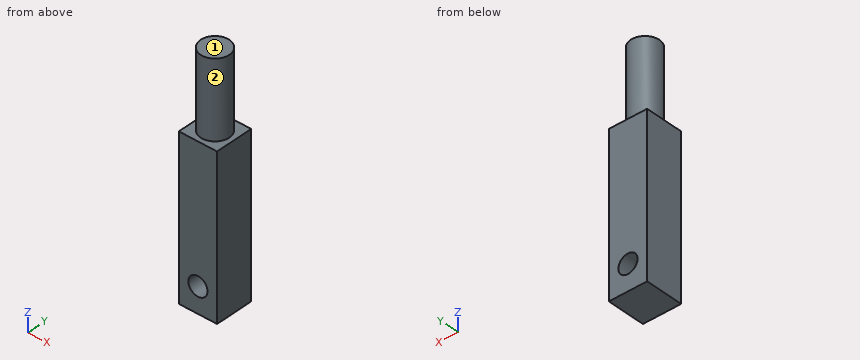
from build123d import *

# Parameters (mm, degrees)
CROQUIS1_W              = 12
CROQUIS1_H              = 12
SALIENTE_EXTRUIR1_DEPTH = 50
CROQUIS2_R              = 4.5
SALIENTE_EXTRUIR2_DEPTH = 24
CROQUIS3_R              = 3
CORTAR_EXTRUIR1_DEPTH   = 76.206382708


with BuildPart() as part:
    # Croquis1 → Saliente-Extruir1 (new body)
    with BuildSketch(Plane.XY):
        Rectangle(CROQUIS1_W, CROQUIS1_H)
    extrude(amount=SALIENTE_EXTRUIR1_DEPTH)

    # Croquis2 → Saliente-Extruir2 (add)
    with BuildSketch(Plane.XY.offset(50)):
        Circle(CROQUIS2_R)
    extrude(amount=SALIENTE_EXTRUIR2_DEPTH)

    # Croquis3 → Cortar-Extruir1 (cut, through all)
    with BuildSketch(Plane(origin=(0, 6, 0), x_dir=(1, 0, 0), z_dir=(0, 1, 0))):
        with Locations(Location((0, -8, 0), (0, 0, 270))):
            Circle(CROQUIS3_R)
    extrude(amount=-CORTAR_EXTRUIR1_DEPTH, mode=Mode.SUBTRACT)


solid = part.part
Can you work these out from the model? Positions are in its coordinate system, mm. Face numbers are marked on the shaded views. A direction names the side the tool comes from. Give positions to 0.01 mm unless a question says otherwise; leave off trailing zeros. Loops run counter-clockwise (first coordinate to the right, second up) from the corner with the lowest first, then second, coordinate; pieces in that order, holes last. Notation, with made-up numbers: (6, 43.5) - (53, 43.5) arc R25 cw to (53, 73.5) - close; hole circle Ø10 at (-5, 29.5). An arc over 180 degrees is marked (long way). One line per item, written item: value.
(1) I need wall thicknesses on line 1 along X through (y, z) = (-2, 8); line 2 along Z through (x, y) = (4, 5); line 3 along Z through (x, y) = (1, 3.25). Which ranges of each line are inside material? Lowest first, please.
Verdict:
line 1: -6 to -3, 3 to 6
line 2: 0 to 50
line 3: 0 to 5.17, 10.83 to 74
(2) If we section it at B-B, the plane x = 0: List the corners of the cut face in (y, z) for me, plus the area to 3 significant figures.
Verdict:
outline: (-6, 0) - (6, 0) - (6, 5) - (-6, 5) - close; (-6, 11) - (6, 11) - (6, 50) - (4.5, 50) - (4.5, 74) - (-4.5, 74) - (-4.5, 50) - (-6, 50) - close
area: 744 mm^2
(3) If we section it at C-C, the plane y = 3.75: List the corners of the cut face in (x, z) for me, plus the area to 3 significant figures.
Verdict:
outline: (-6, 0) - (6, 0) - (6, 50) - (2.49, 50) - (2.49, 74) - (-2.49, 74) - (-2.49, 50) - (-6, 50) - close; hole circle Ø6 at (0, 8)
area: 691 mm^2
(4) If we section it at A-A, the plane z = 8: List the corners of the cut face in (x, y) for me, plus the area to 3 significant figures.
Verdict:
outline: (-6, -6) - (-3, -6) - (-3, 6) - (-6, 6) - close; (3, -6) - (6, -6) - (6, 6) - (3, 6) - close
area: 72.0 mm^2
(5) I'm going to push flat-ended pins straight in: pin 1 (2 mm diameter, centred on x = -4.5, y = 4, fed in from +Z); pin 2 (5 mm diameter, centred on x = 0, z = 8, fed in from -Y); pin 3 (6 mm diameter, centred on y = -3.5, z = 56, fed in from -X); pin 4 (1 mm diameter, centred on x = -3, z = 62, fed in from +Y). Where does each tip first touch, or does it pass through?
Verdict:
pin 1: z = 50
pin 2: through
pin 3: x = -4.47
pin 4: y = 3.74
(6) On a 3-axis mill with a long thin cutter (end or side, diameter ignored), from which of +Z, -Z, +X, -X, +Y, -Y can I reach the whole of each face in a straight line? I mean the marked faces 1 and 2. Say none if no direction works.
Verdict:
face 1: +Z, +X, -X, +Y, -Y
face 2: +Z
(7) If we section it at D-D, the plane z = 57: List the corners of the cut face in (x, y) for me, plus the area to 3 significant figures.
Verdict:
outline: circle Ø9 at (0, 0)
area: 63.6 mm^2
